Design review of the part built by this model. Coordinates are the model's own, in mm. A direction names the side the tool comes from. Give positions to 0.01 mm unless a question says otherwise; leave off trailing zeros. Loops run counter-clockwise (first coordinate to the right, second up) from the corner with the lowest first, then second, coordinate; pieces in that order, holes last. Notation, with made-up numbers: (46, 30) -> (88, 30) arc R22 ccw to (88, 60) -> close; hole circle Ø7 at (-24, 45.25). An arc over 180 degrees is marked (long way). Use a Markdown table: item, result. Add a question column.
1. Add section B-B (y = -5). State the section outline as (x, z) points, and give its area (4 significant figures).
2. For pin 1 Ø6 at (x, y) = (3, 2) entering from +Z; pin 2 Ø0.8 at (x, y) = (-22.5, 7) entering from +Z; pin 3 Ø1.8 at (x, y) = (24.75, -5) entering from -Z; pin 4 Ø1.5 at (y, z) = (5, 20.5) entering from -X, all flat-tipped, find the tip position at first contact; note any pin that passes through.
3. To check wall thickness, follow line 1 (X direction, y = 8.75, z = 9.5); line 2 (X direction, y = 3.5, z = 14.75); line 3 (Z direction, x = -15, y = 4.25). State the ranges of each line that lie inside material, in increasing order.
4. For faces 1 (the flat face through (-23.25, 3, 10)), 2 (the flat face through (22.25, 9, 13)), 3 (the flat face through (-23, -1.5, 8)), list the 3-axis set-ups (+Z, -Z, +X, -X, +Y, -Y) from which the entire face can be reached by the end or side of a thin tool; tool diameter is ignored.
5. Draft analysis for pull direction Y (two halves, no side actions). For faces 4 (the cylindrical face through (-24.936, 9.24, 7.856)), 5 (the flat face through (0, 10, 2)), 6 (the cylindrical face through (-25.487, -4.324, 1.479)), state which applies: pulls with the +Y half, pulls with the -Y half, needs draft (parallel to the pull), parting line crosses it, or undercut.
6. Add section C-C (y = 2). State the section outline as (x, z) points.
```python
from build123d import *

# Parameters (mm, degrees)
F0_W     = 54.5
F0_H     = 20
F0_R     = 1
F1_DEPTH = 3
F2_W     = 5
F2_H     = 1.5
F3_DEPTH = 20
F4_W     = 1
F4_H     = 10
F5_DEPTH = 17.5
F6_SIZE  = 7.5
F8_D     = 1


# Not quite as in the source:
# - a feature names something its author has since deleted; it is built from what else it names


with BuildPart() as f1:
    # F0 (on Top) → F1 (new body)
    with BuildSketch(Plane.XY):
        Rectangle(F0_W, F0_H)
        with Locations((-24.75, -5)):
            Circle(F0_R, mode=Mode.SUBTRACT)
        with Locations((24.75, -5)):
            Circle(F0_R, mode=Mode.SUBTRACT)
        with Locations((-24.75, 5)):
            Circle(F0_R, mode=Mode.SUBTRACT)
        with Locations((24.75, 5)):
            Circle(F0_R, mode=Mode.SUBTRACT)
    extrude(amount=F1_DEPTH)

    # F2 (on face) → F3 (join)
    with BuildSketch(Plane.XY.offset(3)):
        with Locations((-24.75, 9.25)):
            Rectangle(F2_W, F2_H)
        with Locations((24.75, 9.25)):
            Rectangle(F2_W, F2_H)
    extrude(amount=F3_DEPTH)

    # F4 (on face) → F5 (join)
    with BuildSketch(Plane.XY.offset(3)):
        with Locations((-22.75, 3.5)):
            Rectangle(F4_W, F4_H)
        with Locations((22.7855359316, 3.5)):
            Rectangle(F4_W, F4_H)
    extrude(amount=F5_DEPTH)

    # F6
    f6_edges = [f1.edges().sort_by_distance(p)[0] for p in [
        (-22.75, -1.5, 20.5),
        (22.785536, -1.5, 20.5),
    ]]
    chamfer(f6_edges, length=F6_SIZE)

    # F8 (through all)
    with Locations(Plane(origin=(0, 10, 0), x_dir=(-1, 0, 0), z_dir=(0, 1, 0))):
        with Locations((24.8279795051, 8.3445450291), (24.7343406081, 18.3638688177), (-24.8004421592, 8.3445450291), (-24.7068032622, 18.3638688177)):
            Hole(F8_D / 2)


solid = f1.part
```
Taken from the geometry:
| question | item | result |
|---|---|---|
| 1 | outline | (-27.25, 0) -> (-25.75, 0) -> (-25.75, 3) -> (-27.25, 3) -> close; (-23.75, 0) -> (23.75, 0) -> (23.75, 3) -> (-23.75, 3) -> close; (25.75, 0) -> (27.25, 0) -> (27.25, 3) -> (25.75, 3) -> close |
| 1 | area | 151.5 mm^2 |
| 2 | pin 1 | stops at z = 3 |
| 2 | pin 2 | stops at z = 20.5 |
| 2 | pin 3 | passes through |
| 2 | pin 4 | stops at x = -23.25 |
| 3 | line 1 | x = -27.25 to -22.25, 22.25 to 27.25 |
| 3 | line 2 | x = -23.25 to -22.25, 22.29 to 23.29 |
| 3 | line 3 | z = 0 to 3 |
| 4 | face 1 | +Z, -X, -Y |
| 4 | face 2 | +Z, +Y, -Y |
| 4 | face 3 | +Z, +X, -X, -Y |
| 5 | face 4 | needs draft |
| 5 | face 5 | pulls with the +Y half |
| 5 | face 6 | undercut |
| 6 | outline | (-27.25, 0) -> (27.25, 0) -> (27.25, 3) -> (23.29, 3) -> (23.29, 16.5) -> (22.29, 16.5) -> (22.29, 3) -> (-22.25, 3) -> (-22.25, 16.5) -> (-23.25, 16.5) -> (-23.25, 3) -> (-27.25, 3) -> close |
